Verification items for the finished model (mm, model axes). Face numbers are marked on the shaded views. A direction names the side the tool comes from. Give positions to 0.01 mm unless a question says otherwise; leave off trailing zeros. Order: outer loops, then holes, each group sorted by start corner. A loop starts at its lowest first (then second) coordinate and runs counter-clockwise, first axis right, second up. Notation, with made-up numbers: (40, -5) - (50, -5) arc R26 ccw to (50, 9) - close; hole circle Ø7 at (1.25, 69). An arc over 180 degrees is marked (long way). Answer as a JSON object with one key per item and string values.
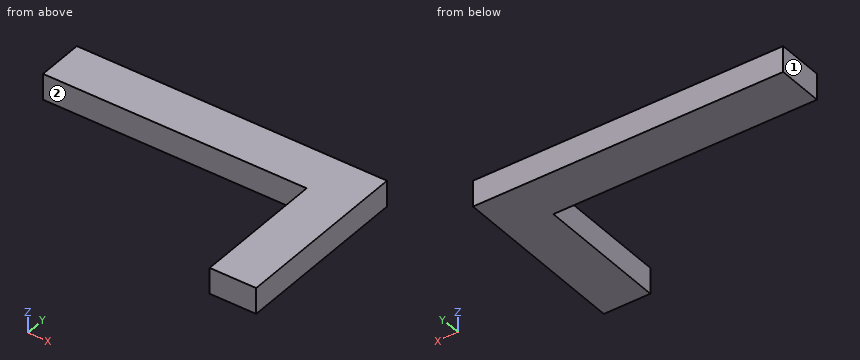
```python
from build123d import *

# Parameters (mm, degrees)
F0_W     = 42.5
F0_H     = 7.5
F0_W_2   = 7.5
F0_H_2   = 21.5
F1_DEPTH = 4.2
F2_DEPTH = 4.2


with BuildPart() as f1:
    # F0 (on Top) → F1 (new body)
    with BuildSketch(Plane.XY):
        with Locations((-3.75, 0)):
            Rectangle(F0_W, F0_H)
        with Locations((21.25, 0)):
            Rectangle(F0_W_2, F0_H)
        with Locations((21.25, -14.5)):
            Rectangle(F0_W_2, F0_H_2)
    extrude(amount=F1_DEPTH)

    # F0 (on Top) → F2 (join)
    with BuildSketch(Plane.XY):
        with Locations((-3.75, 0)):
            Rectangle(F0_W, F0_H)
        with Locations((21.25, 0)):
            Rectangle(F0_W_2, F0_H)
        with Locations((21.25, -14.5)):
            Rectangle(F0_W_2, F0_H_2)
    extrude(amount=F2_DEPTH)


solid = f1.part
```
(1) Access from +Z, -Z, +X, -X, +Y, -Y to the whole of each face (thin tool, end or side, straight path). Record for the marked faces 1 and 2.
Computed values:
{"face 1": "+Z, -Z, -X, +Y, -Y", "face 2": "+Z, -Z, -X, -Y"}
(2) Gauge pin test, flat ends, axial feed: pin 1 Ø1.3 at (y, z) = (-16.5, 2) entering from -X; pin 2 Ø5 at (x, y) = (-0.5, -6.5) entering from +Z. Record the tip position at first contact, or that the pin passes through.
Computed values:
{"pin 1": "stops at x = 17.5", "pin 2": "passes through"}
(3) Material ranges on line 1 along Y through (x, z) = (-4.5, 1.4); line 2 along X through (y, z) = (-5, 1), recorded low to high. Write a range as [from, to].
Computed values:
{"line 1": "y = [-3.75, 3.75]", "line 2": "x = [17.5, 25]"}
(4) Section check B-B (y = -13). Record the cut outline in (x, z), then the cut area to 3 significant figures.
Computed values:
{"outline": "(17.5, 0) - (25, 0) - (25, 4.2) - (17.5, 4.2) - close", "area": "31.5 mm²"}
(5) Section check A-A (z = 0.55). Record the cut outline in (x, y).
Computed values:
{"outline": "(-25, -3.75) - (17.5, -3.75) - (17.5, -25.25) - (25, -25.25) - (25, 3.75) - (-25, 3.75) - close"}
(6) Section check C-C (x = 5.5). Record the cut outline in (y, z), then the cut area to 3 significant figures.
Computed values:
{"outline": "(-3.75, 0) - (3.75, 0) - (3.75, 4.2) - (-3.75, 4.2) - close", "area": "31.5 mm²"}
